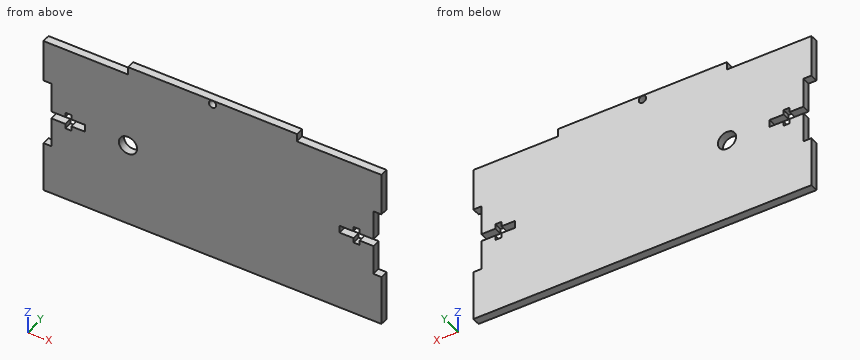
```python
from build123d import *

# Parameters (mm, degrees)
SKETCH1_W           = 127
SKETCH1_H           = 63.5
BOSS_EXTRUDE1_DEPTH = 2.9972
CUT_EXTRUDE1_REACH  = 73.058
SKETCH2_R           = 1.397
SKETCH2_W           = 31.75
SKETCH2_H           = 2.9972
CUT_EXTRUDE2_REACH  = 73.058
SKETCH3_R           = 3.429


with BuildPart() as part:
    # Sketch1 → Boss-Extrude1 (new body)
    with BuildSketch(Plane(origin=(0, 0, 0), x_dir=(1, 0, 0), z_dir=(0, 1, 0))):
        Rectangle(SKETCH1_W, SKETCH1_H)
    extrude(amount=BOSS_EXTRUDE1_DEPTH)

    # Sketch2 → Cut-Extrude1 (cut, up to next)
    with BuildSketch(Plane(origin=(0, 2.9972, 0), x_dir=(1, 0, 0), z_dir=(0, 1, 0)), mode=Mode.PRIVATE) as cut_extrude1_sk1:
        with Locations(Location((0, -30.2514, 0), (0, 0, 90))):
            Circle(SKETCH2_R)
    cut_extrude1_tool1 = extrude(cut_extrude1_sk1.sketch, amount=-CUT_EXTRUDE1_REACH, mode=Mode.PRIVATE) & part.part
    # Sketch2 → Cut-Extrude1 (cut, up to next)
    with BuildSketch(Plane(origin=(0, 2.9972, 0), x_dir=(1, 0, 0), z_dir=(0, 1, 0)), mode=Mode.PRIVATE) as cut_extrude1_sk2:
        with Locations((-47.625, -30.2514)):
            Rectangle(SKETCH2_W, SKETCH2_H)
    cut_extrude1_tool2 = extrude(cut_extrude1_sk2.sketch, amount=-CUT_EXTRUDE1_REACH, mode=Mode.PRIVATE) & part.part
    # Sketch2 → Cut-Extrude1 (cut, up to next)
    with BuildSketch(Plane(origin=(0, 2.9972, 0), x_dir=(1, 0, 0), z_dir=(0, 1, 0)), mode=Mode.PRIVATE) as cut_extrude1_sk3:
        Polygon((-63.5, 12.7), (-60.5028, 12.7), (-60.5028, 1.397), (-55.2958, 1.397), (-55.2958, 3.175), (-53.0098, 3.175), (-53.0098, 1.397), (-47.8028, 1.397), (-47.8028, -1.397), (-53.0098, -1.397), (-53.0098, -3.175), (-55.2958, -3.175), (-55.2958, -1.397), (-60.5028, -1.397), (-60.5028, -12.7), (-63.5, -12.7), align=None)
    cut_extrude1_tool3 = extrude(cut_extrude1_sk3.sketch, amount=-CUT_EXTRUDE1_REACH, mode=Mode.PRIVATE) & part.part
    # Sketch2 → Cut-Extrude1 (cut, up to next)
    with BuildSketch(Plane(origin=(0, 2.9972, 0), x_dir=(1, 0, 0), z_dir=(0, 1, 0)), mode=Mode.PRIVATE) as cut_extrude1_sk4:
        with Locations((47.625, -30.2514)):
            Rectangle(SKETCH2_W, SKETCH2_H)
    cut_extrude1_tool4 = extrude(cut_extrude1_sk4.sketch, amount=-CUT_EXTRUDE1_REACH, mode=Mode.PRIVATE) & part.part
    # Sketch2 → Cut-Extrude1 (cut, up to next)
    with BuildSketch(Plane(origin=(0, 2.9972, 0), x_dir=(1, 0, 0), z_dir=(0, 1, 0)), mode=Mode.PRIVATE) as cut_extrude1_sk5:
        Polygon((60.5028, -1.397), (60.5028, -12.7), (63.5, -12.7), (63.5, 12.7), (60.5028, 12.7), (60.5028, 1.397), (55.2958, 1.397), (55.2958, 3.175), (53.0098, 3.175), (53.0098, 1.397), (47.8028, 1.397), (47.8028, -1.397), (53.0098, -1.397), (53.0098, -3.175), (55.2958, -3.175), (55.2958, -1.397), align=None)
    cut_extrude1_tool5 = extrude(cut_extrude1_sk5.sketch, amount=-CUT_EXTRUDE1_REACH, mode=Mode.PRIVATE) & part.part
    add(cut_extrude1_tool1.solids().sort_by_distance((0, 2.9972, 30.2514))[0], mode=Mode.SUBTRACT)
    add(cut_extrude1_tool2.solids().sort_by_distance((-47.625, 2.9972, 30.2514))[0], mode=Mode.SUBTRACT)
    add(cut_extrude1_tool3.solids().sort_by_distance((-59.14275, 2.9972, 0))[0], mode=Mode.SUBTRACT)
    add(cut_extrude1_tool4.solids().sort_by_distance((47.625, 2.9972, 30.2514))[0], mode=Mode.SUBTRACT)
    add(cut_extrude1_tool5.solids().sort_by_distance((59.14275, 2.9972, 0))[0], mode=Mode.SUBTRACT)

    # Sketch3 → Cut-Extrude2 (cut, up to next)
    with BuildSketch(Plane(origin=(0, 2.9972, 0), x_dir=(1, 0, 0), z_dir=(0, 1, 0)), mode=Mode.PRIVATE) as cut_extrude2_sk1:
        with Locations(Location((-31.75, 0, 0), (0, 0, 270))):
            Circle(SKETCH3_R)
    cut_extrude2_tool1 = extrude(cut_extrude2_sk1.sketch, amount=-CUT_EXTRUDE2_REACH, mode=Mode.PRIVATE) & part.part
    add(cut_extrude2_tool1.solids().sort_by_distance((-31.75, 2.9972, 0))[0], mode=Mode.SUBTRACT)


solid = part.part
```
Input: part model. Units: mm. Frame: model coordinates. Give positions to 0.01 mm unless a question says otherwise; leave off trailing zeros. Order: outer loops, then holes, each group sorted by start corner. A loop starts at its lowest first (then second) coordinate and runs counter-clockwise, first axis right, second up. Notation, with made-up numbers: (57, 17) - (65, 17) arc R26 ccw to (65, 55) - close; hole circle Ø1 at (-13, -38). An arc over 180 degrees is marked (long way). Put each result on its own line as item: value.
Item 1: Ray query, L1, parallel to X at y = 1.6, z = 0; L2, parallel to X at y = 1.95, z = 11; L3, parallel to Z at x = -43.5, y = 1.8. Return the intervals inside material, ascending. Write a range as from..to.
Found:
L1: x = -47.8..-35.18, -28.32..47.8
L2: x = -60.5..60.5
L3: z = -31.75..28.75
Item 2: Section query A-A, the plane z = 0. Return loops of the section in (x, y).
Found:
outline: (-47.8, 0) - (-35.18, 0) - (-35.18, 3) - (-47.8, 3) - close; (-28.32, 0) - (47.8, 0) - (47.8, 3) - (-28.32, 3) - close
Item 3: Section query B-B, the plane x = 0. Return loops of the section in (y, z), then the cut area to 3 significant figures.
Found:
outline: (0, -31.75) - (3, -31.75) - (3, 28.85) - (0, 28.85) - close; (0, 31.65) - (3, 31.65) - (3, 31.75) - (0, 31.75) - close
area: 182 mm^2
Item 4: Contact query for flat-ended pins moving along their axis: pin 1 (0.5 mm diameter, centred on y = 2, z = -2.5, fed in from +X); pin 2 (1.5 mm diameter, centred on x = -50, y = 2, fed in from +Z); pin 3 (1.5 mm diameter, centred on y = 1, z = 30, fed in from +X). Output: stop coordinate, or through.
Found:
pin 1: stops at x = 60.5
pin 2: stops at z = 28.75
pin 3: stops at x = 31.75
Item 5: Section query D-D, the plane z = 11.5. Return loops of the section in (x, y), then the cut area to 3 significant figures.
Found:
outline: (-60.5, 0) - (60.5, 0) - (60.5, 3) - (-60.5, 3) - close
area: 363 mm^2
Item 6: Section query C-C, the plane y = 0.65. Count the separate pieces of the cut face and the enclosed holes in it, then the cut area to 3 significant figures.
Found:
separate pieces: 1
enclosed holes: 2
area: 7,590 mm^2
